CAD build for the part. Positions are in the model's coordinates, mm. Face numbers are marked on the shaded views. A direction names the side the tool comes from. Give positions to 0.01 mm unless a question says otherwise; leave off trailing zeros. Loops run counter-clockwise (first coordinate to the right, second up) from the corner with the lowest first, then second, coordinate; pieces in that order, holes last. Notation, with made-up numbers: (-4.5, 53.5) -> (4.5, 53.5) arc R35 ccw to (4.5, 88.5) -> close; hole circle Ø1 at (85, 38.25). An arc over 180 degrees is marked (long way). Use one line per item in the form item = value.
```python
from build123d import *

# Parameters (mm, degrees)
SKETCH1_W                                    = 48
SKETCH1_H                                    = 48
SKETCH1_W_2                                  = 42
SKETCH1_H_2                                  = 42
BOSS_EXTRUDE1_DEPTH                          = 65
SKETCH3_W                                    = 75
SKETCH3_H                                    = 75
BOSS_EXTRUDE2_DEPTH                          = 5
SKETCH8_W                                    = 75
SKETCH8_H                                    = 75
SKETCH8_W_2                                  = 42
SKETCH8_H_2                                  = 42
BOSS_EXTRUDE3_DEPTH                          = 5.047079132
FILLET1_R                                    = 2
CBORE_FOR_M6_HEX_SOCKET_HEAD_CAP_SCR_2_COUNT = 2
CBORE_FOR_M6_HEX_SOCKET_HEAD_CAP_SCR_2_PITCH = 50
CBORE_FOR_M6_HEX_SOCKET_HEAD_CAP_SCR_3_COUNT = 2
CBORE_FOR_M6_HEX_SOCKET_HEAD_CAP_SCR_3_PITCH = 61.5
CBORE_FOR_M6_HEX_SOCKET_HEAD_CAP_SCR_4_COUNT = 2
CBORE_FOR_M6_HEX_SOCKET_HEAD_CAP_SCR_4_PITCH = 79.260645973


with BuildPart() as part:
    # Sketch1 → Boss-Extrude1 (new body)
    with BuildSketch(Plane(origin=(0, 0, 0), x_dir=(0, 1, 0), z_dir=(0, 0, 1))):
        with Locations((-1.048003873, 6.146094376)):
            Rectangle(SKETCH1_W, SKETCH1_H)
        with Locations((-1.048003873, 6.146094376)):
            Rectangle(SKETCH1_W_2, SKETCH1_H_2, mode=Mode.SUBTRACT)
    extrude(amount=BOSS_EXTRUDE1_DEPTH)

    # Sketch3 → Boss-Extrude2 (add)
    with BuildSketch(Plane(origin=(0, 0, 0), x_dir=(1, 0, 0), z_dir=(0, 0, -1))):
        with Locations((-6.146094376, 1.048003873)):
            Rectangle(SKETCH3_W, SKETCH3_H)
    extrude(amount=BOSS_EXTRUDE2_DEPTH)

    # Sketch8 → Boss-Extrude3 (add)
    with BuildSketch(Plane.XY):
        with Locations((-6.146094376, -1.048003873)):
            Rectangle(SKETCH8_W, SKETCH8_H)
        with Locations((-6.146094376, -1.048003873)):
            Rectangle(SKETCH8_W_2, SKETCH8_H_2, mode=Mode.SUBTRACT)
    extrude(amount=BOSS_EXTRUDE3_DEPTH)

    # Fillet1
    fillet1_edges = [part.edges().sort_by_distance(p)[0] for p in [
        (17.853905624, 22.951996127, 35.023539566),
        (17.853905624, -25.048003873, 35.023539566),
        (-30.146094376, -25.048003873, 35.023539566),
        (-30.146094376, 22.951996127, 35.023539566),
        (-43.646094376, -38.548003873, 0.023539566),
        (31.353905624, -38.548003873, 0.023539566),
        (31.353905624, 36.451996127, 0.023539566),
        (-43.646094376, 36.451996127, 0.023539566),
    ]]
    fillet(fillet1_edges, radius=FILLET1_R)

    # Sketch15 → CBORE for M6 Hex Socket Head Cap Screw2 (revolve, cut)
    with BuildSketch(Plane(origin=(-36.896094376, 23.951996127, 5.047079132), x_dir=(0, -1, 0), z_dir=(1, 0, 0))):
        Polygon((0, 0), (0, 10.047079132), (3.3, 10.047079132), (3.3, 6.4), (5.5, 6.4), (5.5, 0.025), (5.525, 0), align=None)
    cbore_for_m6_hex_socket_head_cap_screw2 = revolve(axis=Axis((-36.896094376, 23.951996127, 11.397079132), (0, 0, -1)), mode=Mode.SUBTRACT)

    # CBORE for M6 Hex Socket Head Cap Scr 2: CBORE for M6 Hex Socket Head Cap Screw2 ×2
    with Locations(*[(0, -i * CBORE_FOR_M6_HEX_SOCKET_HEAD_CAP_SCR_2_PITCH, 0) for i in range(1, CBORE_FOR_M6_HEX_SOCKET_HEAD_CAP_SCR_2_COUNT)]):
        add(cbore_for_m6_hex_socket_head_cap_screw2, mode=Mode.SUBTRACT)

    # CBORE for M6 Hex Socket Head Cap Scr 3: CBORE for M6 Hex Socket Head Cap Screw2 ×2
    with Locations(*[(i * CBORE_FOR_M6_HEX_SOCKET_HEAD_CAP_SCR_3_PITCH, 0, 0) for i in range(1, CBORE_FOR_M6_HEX_SOCKET_HEAD_CAP_SCR_3_COUNT)]):
        add(cbore_for_m6_hex_socket_head_cap_screw2, mode=Mode.SUBTRACT)

    # CBORE for M6 Hex Socket Head Cap Scr 4: CBORE for M6 Hex Socket Head Cap Screw2 ×2
    with Locations(*[Vector(0.7759210039901774, -0.63083008454486, 0) * (i * CBORE_FOR_M6_HEX_SOCKET_HEAD_CAP_SCR_4_PITCH) for i in range(1, CBORE_FOR_M6_HEX_SOCKET_HEAD_CAP_SCR_4_COUNT)]):
        add(cbore_for_m6_hex_socket_head_cap_screw2, mode=Mode.SUBTRACT)


solid = part.part
```
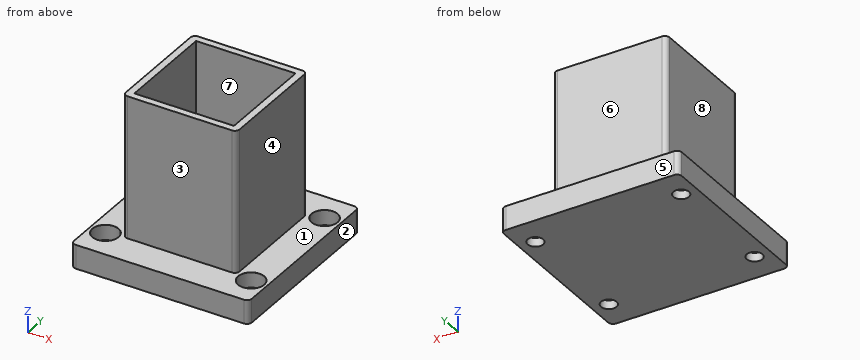
1. Tool access for the marked faces 1, 2, 3, 4 and 5: list every direction of +Z, -Z, +X, -X, +Y, -Y with a clear straight run to the whole face (end or side of a thin tool).
Result sheet:
face_1 = +Z
face_2 = +Z, -Z, +X, +Y, -Y
face_3 = +Z, +X, -X, -Y
face_4 = +Z, +X, +Y, -Y
face_5 = +Z, -Z, +X, -X, +Y
2. Mould opens along Y. For the marked faces 6, 7 and 8 say: pulls with the +Y half, pulls with the -Y half, needs draft (parallel to the pull), parting line crosses it, or undercut.
Result sheet:
face_6 = pulls with the +Y half
face_7 = undercut
face_8 = needs draft
3. Cut at C-C, the plane y = -15.5. Write the cut outline in (x, z).
Result sheet:
outline = (-43.65, -5) -> (31.35, -5) -> (31.35, 5.05) -> (17.85, 5.05) -> (17.85, 65) -> (14.85, 65) -> (14.85, 0) -> (-27.15, 0) -> (-27.15, 65) -> (-30.15, 65) -> (-30.15, 5.05) -> (-43.65, 5.05) -> close
4. Cut at B-B, the plane x = -8.5. Write the cut outline in (y, z).
Result sheet:
outline = (-38.55, -5) -> (36.45, -5) -> (36.45, 5.05) -> (22.95, 5.05) -> (22.95, 65) -> (19.95, 65) -> (19.95, 0) -> (-22.05, 0) -> (-22.05, 65) -> (-25.05, 65) -> (-25.05, 5.05) -> (-38.55, 5.05) -> close
5. Cut at A-A, the plane z = 32. Write the cut outline in (x, y), then the cut area to 3 significant figures.
Result sheet:
outline = (-30.15, -23.05) arc R2 ccw to (-28.15, -25.05) -> (15.85, -25.05) arc R2 ccw to (17.85, -23.05) -> (17.85, 20.95) arc R2 ccw to (15.85, 22.95) -> (-28.15, 22.95) arc R2 ccw to (-30.15, 20.95) -> close; hole (-27.15, -22.05) -> (14.85, -22.05) -> (14.85, 19.95) -> (-27.15, 19.95) -> close
area = 537 mm^2
6. Drill centre lines: line 1 (Y direction, x = -7.5, z = 9); line 2 (X direction, y = 2, z = 38); line 3 (Y direction, x = 6, z = 4.5). Where is each one in solid material? Low to high.
Result sheet:
line_1 = -25.05 to -22.05, 19.95 to 22.95
line_2 = -30.15 to -27.15, 14.85 to 17.85
line_3 = -38.55 to -22.05, 19.95 to 36.45
7. Drop flat-ended pins along their axis: P1, Ø5, axis at y = -2.5, z = 20, coming from the +X side; P2, Ø1.5, axis at x = -23.5, y = 17.5, coming from the +Z side; P3, Ø10, axis at y = 12, z = 44.5, coming from the -X side. Give the stop position or say it passes through.
Result sheet:
P1 = 17.85
P2 = 0
P3 = -30.15
